from build123d import *

# Parameters (mm, degrees)
F1_DEPTH = 30
F2_R     = 8.4944799553
F2_R_2   = 6.50875
F3_DEPTH = 25
F4_R     = 11.8009083685
F4_R_2   = 6.50875
F5_DEPTH = 25


with BuildPart() as f1:
    # F0 (on Front) → F1 (new body)
    with BuildSketch(Plane.XZ):
        Polygon((-2.3517715285, 45.0519641835), (-15.7493199024, 58.4674571651), (-66.1214962602, -28.7797115743), (63.1061792374, -28.7797115743), (63.1061792374, -2.0140784685), (-29.5253639234, -2.0140784685), align=None)
    extrude(amount=F1_DEPTH)

    # F2 (on face) → F3 (join)
    with BuildSketch(Plane(origin=(21.3485022284, 0, 21.3199464014), x_dir=(0, 1, 0), z_dir=(0.7075798534, 0, 0.7066333923))):
        with Locations((-15, 43.0195463119)):
            Circle(F2_R)
        with Locations((-15, 43.0195463119)):
            Circle(F2_R_2, mode=Mode.SUBTRACT)
    extrude(amount=F3_DEPTH)

    # F4 (on face) → F5 (join)
    with BuildSketch(Plane.YZ.offset(63.1061792374)):
        with Locations((-15, -15.3968950214)):
            Circle(F4_R)
        with Locations((-15, -15.3968950214)):
            Circle(F4_R_2, mode=Mode.SUBTRACT)
    extrude(amount=F5_DEPTH)


solid = f1.part
Geometry check sheet. Reference: the model listing, model coordinates, mm. A direction names the side the tool comes from. Round coordinates to 2 decimals unless told otherwise and drop trailing zeros. Order: outer loops, then holes, each group sorted by start corner. A loop starts at its lowest first (then second) coordinate and runs counter-clockwise, first axis right, second up. Notation, with made-up numbers: (-18.5, -15.75) -> (-8.5, -15.75) arc R12 ccw to (-8.5, -7.75) -> close; hole circle Ø10 at (87, 29.25). An arc over 180 degrees is marked (long way). Use one line per item in the form item = value.
1. Set-up check for faces 4 (the face through (-2, -15, -28.78)), 5 (the face through (-8.99, -14.91, 51.7)), 6 (the face through (17, -15, -2.014)), 7 (the face through (88.106, -10, -20)), 8 (the face through (63.106, -15, -15)): record each of +Z, -Z, +X, -X, +Y, -Y from which the full face is reachable in a straight line by a thin tool's end or side.
Working result:
face_4 = -Z, +X, -X, +Y, -Y
face_5 = none
face_6 = +X, +Y, -Y
face_7 = +Z, -Z, +X, +Y, -Y
face_8 = +X
2. Cross-section at A-A, the plane x = -21. Enter the section's corners in (y, z), plus the area to 3 significant figures.
Working result:
outline = (-30, -28.78) -> (0, -28.78) -> (0, -2.01) -> (-30, -2.01) -> close; (-30, 12.75) -> (0, 12.75) -> (0, 49.37) -> (-30, 49.37) -> close
area = 1,900 mm^2
3. Cross-section at D-D, the plane z = 8. Enter the section's corners in (x, y).
Working result:
outline = (-44.89, -30) -> (-23.74, -30) -> (-23.74, 0) -> (-44.89, 0) -> close
4. Cross-section at C-C, the plane x = 31.5. Enter the section's corners in (y, z).
Working result:
outline = (-30, -28.78) -> (0, -28.78) -> (0, -2.01) -> (-30, -2.01) -> close
5. Cross-section at B-B, the plane y = -15. Enter the section's corners in (x, z).
Working result:
outline = (-66.12, -28.78) -> (63.11, -28.78) -> (63.11, -27.2) -> (88.11, -27.2) -> (88.11, -21.91) -> (63.11, -21.91) -> (63.11, -8.89) -> (88.11, -8.89) -> (88.11, -3.6) -> (63.11, -3.6) -> (63.11, -2.01) -> (-29.53, -2.01) -> (-2.35, 45.05) -> (-3.05, 45.75) -> (14.64, 63.42) -> (13.24, 64.82) -> (-4.45, 47.15) -> (-13.65, 56.37) -> (4.04, 74.03) -> (2.64, 75.44) -> (-15.05, 57.77) -> (-15.75, 58.47) -> close
6. Scan lines: line 1 along Z through (x, y) = (80, -15); line 2 along Z through (x, y) = (39.5, -18.75); line 3 along Z through (x, y) = (-23, -25.75). Record each from-to range of solid material in increasing order. Write a range as from..to.
Working result:
line_1 = -27.2..-21.91, -8.89..-3.6
line_2 = -28.78..-2.01
line_3 = -28.78..-2.01, 9.29..45.91
7. Go/stop test with flat-tipped pins: pin 1 (10.5 mm diameter, centred on y = -15, z = -15.4, fed in from +X); pin 2 (10 mm diameter, centred on y = -7.5, z = 48, fed in from -X); pin 3 (3 mm diameter, centred on y = -8.5, z = 2, fed in from +X). Record where each tip stops, or that it passes through.
Working result:
pin_1 = 63.11
pin_2 = -24.68
pin_3 = -26.34
8. Mould release check, pull along Z, two halves, no side actions. Record for faces 1 (the face through (13.06, -12.52, 65)), 2 (the face through (-2, 0, -4)), 3 (the face through (-0.532, -21.502, 60.671)): pulls with the +Z half, pulls with the -Z half, needs draft (parallel to the pull), parting line crosses it, or undercut.
Working result:
face_1 = pulls with the +Z half
face_2 = needs draft
face_3 = undercut
